Build history of the part. All positions in model axes, mm. A direction names the side the tool comes from. Round coordinates to 2 decimals unless told otherwise and drop trailing zeros. Loops run counter-clockwise (first coordinate to the right, second up) from the corner with the lowest first, then second, coordinate; pieces in that order, holes last. Notation, with made-up numbers: (-26.75, -38.5) - (-0.75, -38.5) arc R7 cw to (-0.75, -32.5) - close; hole circle Ø9 at (54, -35.5). An arc over 180 degrees is marked (long way). Use one line per item in the form item = value. Start each with the question number.
Q1. Drill centre lines: line 1 (Y direction, x = -9.5, z = 1.1); line 2 (Y direction, x = -11.5, z = 0.7); line 3 (Y direction, x = 2.55, z = 1.15). Where is each one in solid material? Low to high.
Q2. Saw through at B-B (x = 2.55). Give the cut face in (y, z), then the cut area to 3 significant figures.
Q3. Saw through at D-D (y = -9). Give the cut face in (x, z).
Q4. 3-axis set-ups, long thin cutter, end or side, ignore diameter. For faces 1 (the face through (-2.5, 0.2, 2.5)), 2 (the face through (16, -16.07, 1.48)): which of +Z, -Z, +X, -X, +Y, -Y reach the whole face in a straight line?
Q5. Mould opens along X. For faces 3 (the face through (-16, 16.07, 0.99)), 4 (the face through (7, 0, 3)), 5 (the face through (-10.04, 7.56, 0.99)), 6 (the face through (1.44, 11.91, 1.48)) say: released by +X, released by -X, zero draft, split by the parting line, or undercut.
Q6. Pin check, flat tips, straight feed: pin 1 (4.5 mm diameter, centred on x = -8.5, y = -5, fed in from +Z); pin 2 (2.5 mm diameter, centred on x = 2.55, y = 10.9, fed in from -Z); pin 3 (1.5 mm diameter, centred on x = 13.5, z = 0.5, fed in from +Y). Stop position of each tip, or through.
Q7. Saw through at A-A (y = 10). Give the cut face in (x, z), then the cut area to 3 significant figures.
Q8. Saw through at C-C (z = 0.8). Give the cut face in (x, y).
```python
from build123d import *

# Parameters (mm, degrees)
F0_R     = 1.5
F1_DEPTH = 3
F0_R_2   = 2.5
F2_DEPTH = 2


# Not quite as in the source:
# - a feature of the source that left no trace in its solid (it failed there, or was rolled back) is left out


with BuildPart() as f1:
    # F0 (on Top) → F1 (new body)
    with BuildSketch(Plane.XY):
        with BuildLine():
            Line((-2.5, -17.5), (12.5, -17.5))
            ThreePointArc((12.5, -17.5), (16.0355339059, -16.0355339059), (17.5, -12.5))
            Line((17.5, -12.5), (17.5, 12.5))
            ThreePointArc((17.5, 12.5), (16.0355339059, 16.0355339059), (12.5, 17.5))
            Line((12.5, 17.5), (-2.5, 17.5))
            Line((-2.5, 17.5), (-2.5, -17.5))
        make_face()
        with Locations((12.45, -10.9)):
            Circle(F0_R, mode=Mode.SUBTRACT)
        with Locations((2.55, 10.9)):
            Circle(F0_R, mode=Mode.SUBTRACT)
    extrude(amount=F1_DEPTH)

    # F0 (on Top) → F2 (join)
    with BuildSketch(Plane.XY):
        with BuildLine():
            Line((-12.5, -17.5), (-2.5, -17.5))
            Line((-2.5, -17.5), (-2.5, 17.5))
            Line((-2.5, 17.5), (-12.5, 17.5))
            ThreePointArc((-12.5, 17.5), (-16.0355339059, 16.0355339059), (-17.5, 12.5))
            Line((-17.5, 12.5), (-17.5, -12.5))
            ThreePointArc((-17.5, -12.5), (-16.0355339059, -16.0355339059), (-12.5, -17.5))
        make_face()
        with Locations((-9.5, -10)):
            Circle(F0_R_2, mode=Mode.SUBTRACT)
        with Locations((-9.5, 10)):
            Circle(F0_R_2, mode=Mode.SUBTRACT)
    extrude(amount=F2_DEPTH)


solid = f1.part
```
Report:
q1.line_1 = -17.5 to -12.5, -7.5 to 7.5, 12.5 to 17.5
q1.line_2 = -17.5 to -11.5, -8.5 to 8.5, 11.5 to 17.5
q1.line_3 = -17.5 to 9.4, 12.4 to 17.5
q2.outline = (-17.5, 0) - (9.4, 0) - (9.4, 3) - (-17.5, 3) - close; (12.4, 0) - (17.5, 0) - (17.5, 3) - (12.4, 3) - close
q2.area = 96.0 mm²
q3.outline = (-17.5, 0) - (-11.79, 0) - (-11.79, 2) - (-17.5, 2) - close; (-7.21, 0) - (17.5, 0) - (17.5, 3) - (-2.5, 3) - (-2.5, 2) - (-7.21, 2) - close
q4.face_1 = +Z, -X, +Y, -Y
q4.face_2 = +Z, -Z, +X, -Y
q5.face_3 = released by -X
q5.face_4 = zero draft
q5.face_5 = undercut
q5.face_6 = undercut
q6.pin_1 = 2
q6.pin_2 = through
q6.pin_3 = 17.49
q7.outline = (-17.5, 0) - (-12, 0) - (-12, 2) - (-17.5, 2) - close; (-7, 0) - (1.35, 0) - (1.35, 3) - (-2.5, 3) - (-2.5, 2) - (-7, 2) - close; (3.75, 0) - (17.5, 0) - (17.5, 3) - (3.75, 3) - close
q7.area = 72.8 mm²
q8.outline = (-17.5, -12.5) arc R5 ccw to (-12.5, -17.5) - (12.5, -17.5) arc R5 ccw to (17.5, -12.5) - (17.5, 12.5) arc R5 ccw to (12.5, 17.5) - (-12.5, 17.5) arc R5 ccw to (-17.5, 12.5) - close; hole circle Ø5 at (-9.5, -10); hole circle Ø5 at (-9.5, 10); hole circle Ø3 at (2.55, 10.9); hole circle Ø3 at (12.45, -10.9)
